```python
from build123d import *

# Parameters (mm, degrees)
FILLET1_R       = 0.254
HEX_2_DEPTH     = 1.6256
THDSCHPAT_COUNT = 16
THDSCHPAT_PITCH = 0.74422


with BuildPart() as part:
    # BodySke → Base-Revolve (revolve)
    with BuildSketch(Plane.XY):
        Polygon((0, 0), (0, 2.5146), (0.3556, 2.8702), (3.5052, 2.8702), (3.5052, 1.7526), (15.73276, 1.7526), (16.2052, 1.28016), (16.2052, 0), align=None)
    revolve(axis=Axis((-31.75, 0, 0), (1, 0, 0)))

    # Fillet1
    fillet1_edges = [part.edges().sort_by_distance(p)[0] for p in [
        (3.5052, -1.7526, 0),
    ]]
    fillet(fillet1_edges, radius=FILLET1_R)

    # Sketch2 → Hex-PreBroach (revolve, cut)
    with BuildSketch(Plane.XY):
        Polygon((0, 1.3843), (1.6256, 1.3843), (2.424825978, 0), (0, 0), align=None)
    revolve(axis=Axis((0, 0, 0), (1, 0, 0)), mode=Mode.SUBTRACT)

    # Sketch3 → Hex 2 (cut)
    with BuildSketch(Plane(origin=(0, 0, 0), x_dir=(0, 0.5, 0.866025404), z_dir=(-1, 0, 0))):
        Polygon((0.799225978, 1.3843), (-0.799225978, 1.3843), (-1.598451955, 0), (-0.799225978, -1.3843), (0.799225978, -1.3843), (1.598451955, 0), align=None)
    extrude(amount=-HEX_2_DEPTH, mode=Mode.SUBTRACT)

    # ThdSchSke → ThreadSchematic (revolve, cut)
    with BuildSketch(Plane.XY):
        Polygon((4.29768, -1.28016), (3.966873951, -1.7526), (3.966873951, -2.19075), (4.628486049, -2.19075), (4.628486049, -1.7526), align=None)
    threadschematic = revolve(axis=Axis((-3.175, 0, 0), (1, 0, 0)), mode=Mode.SUBTRACT)

    # ThdSchPat: ThreadSchematic ×16
    with Locations(*[(i * THDSCHPAT_PITCH, 0, 0) for i in range(1, THDSCHPAT_COUNT)]):
        add(threadschematic, mode=Mode.SUBTRACT)


solid = part.part
```
The listing builds one solid part. Answer for the finished solid, in the listing's coordinates (mm). Coordinates: 2 decimals unless noted, no trailing zeros. Return JSON: item names as keys, results as strings. Group by question number.
1. Determine the mould class of faces 1 (the cylindrical face through (1.952, -2.278, -1.746)), 2 (the flat face through (0.801, 1.204, -0.682)) for opening direction Y: released by +Y, released by -Y, zero draft, split by the parting line, or undercut.
2. Given pin 1 (2 mm diameter, centred on x = 6.5, y = 2, fed in from +Z); pin 2 (0.6 mm diameter, centred on y = -0.5, z = 1, fed in from -X); pin 3 (3 mm diameter, centred on x = 7, z = -0.5, fed in from -Y), each flat-ended and moving along its own axis, determine where each tip first touches the part or whether it passes through.
3. Straight lines are drawn through the part: L1, parallel to X at y = 2.25, z = -1.05; L2, parallel to Y at x = 2.5, z = -2.05; L3, parallel to Y at x = 9.75, z = 0.25. For each, find the intervals that lie inside material, in ascending order.
Ans:
{
 "1": {"face 1": "split by the parting line", "face 2": "undercut"},
 "2": {"pin 1": "z = 1.41", "pin 2": "x = 1.63", "pin 3": "y = -1.75"},
 "3": {"L1": "0 to 3.51", "L2": "-2.01 to 2.01", "L3": "-1.61 to 1.61"}
}
